Can you work these out from the model? Positions are in its coordinate system, mm. A direction names the side the tool comes from. Give positions to 0.01 mm unless a question says otherwise; leave off trailing zeros. Write each loop counter-clockwise with the first axis right and the second up, starting at its lowest first coordinate (ties: lowest second). Pieces come first, ordered by that corner, then holes.
1. Suppose I cut it at B-B (x = 0). Please give me the cut outline in (y, z), and give its area (3 significant figures).
2. On a 3-axis mill with a long thin cutter (end or side, diameter ignored), from which of +Z, -Z, +X, -X, +Y, -Y can I reach the whole of each face in a straight line? I mean faces 3 (the flat face through (38.6, 0.4, -19.9)), 4 (the cylindrical face through (-20.96, -16.56, -26.84)), 5 (the flat face through (-20.625, -2, -38)). Say none if no direction works.
3. If I drill on probe 1 along X at (y, z) = (-15, -34.1) (3 decimals); probe 2 along Y at (x, z) = (-16, -33); probe 3 along Y at (x, z) = (16, -27.5), over which ranges is the centre line in solid material (lowest first)?
4. Thinking about a two-plate mould opening in X: for faces 1 (the flat face through (32.35, 0.39, -13.32)), 2 (the cylindrical face through (32.097, 0.147, -14.115)), which applies, pulls with the +X half, pulls with the -X half, needs draft (parallel to the pull), parting line crosses it, or undercut?
5. Suppose I cut it at A-A (z = 0). Please give me the cut outline in (x, y), and give its area (3 significant figures).
6. Suppose I cut it at D-D (y = 8.5). Please give me the cut outline in (x, z) (1 decimal), and give its area (3 significant figures).
7. I'm going to push flat-ended pins straight in: pin 1 (7 mm diameter, centred on x = -16, y = -15, fed in from -Z); pin 2 (4 mm diameter, centred on x = 10.5, y = -6, fed in from +Z); pin 3 (10 mm diameter, centred on y = -12, z = 20.5, fed in from +X); pin 4 (13.5 mm diameter, centred on x = -16, y = -15, fed in from -Z). Where does each tip first touch, or does it pass through?
8. Suppose I cut it at C-C (x = 16). Please give me the cut outline in (y, z).
```python
from build123d import *

# Parameters (mm, degrees)
BOSS_EXTRUDE1_DEPTH                            = 27.5
CBORE_FOR_M3_SBHCS1_D                          = 3.4
CBORE_FOR_M3_SBHCS1_DEPTH                      = 20.0000108
CBORE_FOR_M3_SBHCS1_CBORE_D                    = 6.7
CBORE_FOR_M3_SBHCS1_CBORE_DEPTH                = 1.65
CBORE_FOR_M3_SBHCS1_TIP                        = 1.021463052
SKETCH4_W                                      = 41.25
SKETCH4_H                                      = 6.157842489
BOSS_EXTRUDE2_DEPTH                            = 4.5
CSK_FOR_M5_FLAT_HEAD_MACHINE_SCREW1_AT_2_COUNT = 2
CSK_FOR_M5_FLAT_HEAD_MACHINE_SCREW1_AT_2_PITCH = 32
CSK_FOR_M5_FLAT_HEAD_MACHINE_SCREW1_AT_3_COUNT = 2
CSK_FOR_M5_FLAT_HEAD_MACHINE_SCREW1_AT_3_PITCH = 43.863424399
CSK_FOR_M5_FLAT_HEAD_MACHINE_SCREW1_AT_4_COUNT = 2
CSK_FOR_M5_FLAT_HEAD_MACHINE_SCREW1_AT_4_PITCH = 30
CUT_EXTRUDE1_REACH                             = 81.852
CUT_EXTRUDE1_END_RADIUS                        = 30.1625
SKETCH13_R                                     = 5.2


with BuildPart() as part:
    # Sketch1 → Boss-Extrude1 (new, symmetric)
    with BuildSketch(Plane(origin=(0, 0, 0), x_dir=(1, 0, 0), z_dir=(0, 1, 0))):
        with BuildLine():
            Line((-25.625, 41.495342489), (-25.625, 21.324827813))
            ThreePointArc((-25.625, 21.324827813), (-5.163493362, -32.935197624), (30.921632796, 12.45959596))
            Line((30.921632796, 12.45959596), (39.848528412, 17.823415986))
            Line((39.848528412, 17.823415986), (37.273338038, 22.109252489))
            Line((37.273338038, 22.109252489), (28.701665031, 16.95887174))
            Line((28.701665031, 16.95887174), (28.843705147, 8.821398963))
            ThreePointArc((28.843705147, 8.821398963), (-27.915992451, -11.422511622), (26.75426667, 13.927872098))
            Line((26.75426667, 13.927872098), (26.647715613, 20.032178086))
            Line((26.647715613, 20.032178086), (35.371714531, 25.274085476))
            Line((35.371714531, 25.274085476), (32.281486081, 30.41708928))
            Line((32.281486081, 30.41708928), (23.557487163, 25.17518189))
            Line((23.557487163, 25.17518189), (20.982296789, 29.461018394))
            Line((20.982296789, 29.461018394), (29.706295707, 34.702925784))
            Line((29.706295707, 34.702925784), (25.625, 41.495342489))
            Line((25.625, 41.495342489), (20.625, 41.495342489))
            Line((20.625, 41.495342489), (20.625, 35.3375))
            Line((20.625, 35.3375), (-20.625, 35.3375))
            Line((-20.625, 35.3375), (-20.625, 41.495342489))
            Line((-20.625, 41.495342489), (-25.625, 41.495342489))
        make_face()
    extrude(amount=BOSS_EXTRUDE1_DEPTH, both=True)

    # CBORE for M3 SBHCS1
    with Locations(Plane(origin=(2.701817631, 0, 4.496579649), x_dir=(0.8571673007021098, 0, -0.5150380749100585), z_dir=(0.5150380749100585, 0, 0.8571673007021098))):
        with Locations((38.129386114, 20), (38.129386114, 0), (38.129386114, -20)):
            CounterBoreHole(CBORE_FOR_M3_SBHCS1_D / 2, CBORE_FOR_M3_SBHCS1_CBORE_D / 2, CBORE_FOR_M3_SBHCS1_CBORE_DEPTH, depth=CBORE_FOR_M3_SBHCS1_DEPTH)
            with Locations((0, 0, -(CBORE_FOR_M3_SBHCS1_DEPTH + CBORE_FOR_M3_SBHCS1_TIP / 2))):  # 118° drill point
                Cone(0, CBORE_FOR_M3_SBHCS1_D / 2, CBORE_FOR_M3_SBHCS1_TIP, mode=Mode.SUBTRACT)

    # Sketch4 → Boss-Extrude2 (add)
    with BuildSketch(Plane.XZ.offset(-27.5)):
        with Locations((0, -38.416421245)):
            Rectangle(SKETCH4_W, SKETCH4_H)
    extrude(amount=BOSS_EXTRUDE2_DEPTH)

    # Sketch12 → CSK for M5 Flat Head Machine Screw1 (revolve, cut)
    with BuildSketch(Plane(origin=(-16, 15, -30.1625), x_dir=(0, -1, 0), z_dir=(1, 0, 0))):
        Polygon((0, 0), (0, 11.332842489), (2.75, 11.332842489), (2.75, 2.45), (5.2, 0), align=None)
    csk_for_m5_flat_head_machine_screw1 = revolve(axis=Axis((-16, 15, -23.8125), (0, 0, -1)), mode=Mode.SUBTRACT)

    # CSK for M5 Flat Head Machine Screw1 at 2: CSK for M5 Flat Head Machine Screw1 ×2
    with Locations(*[(i * CSK_FOR_M5_FLAT_HEAD_MACHINE_SCREW1_AT_2_PITCH, 0, 0) for i in range(1, CSK_FOR_M5_FLAT_HEAD_MACHINE_SCREW1_AT_2_COUNT)]):
        add(csk_for_m5_flat_head_machine_screw1, mode=Mode.SUBTRACT)

    # CSK for M5 Flat Head Machine Screw1 at 3: CSK for M5 Flat Head Machine Screw1 ×2
    with Locations(*[Vector(0.7295372041400853, -0.6839411288813297, 0) * (i * CSK_FOR_M5_FLAT_HEAD_MACHINE_SCREW1_AT_3_PITCH) for i in range(1, CSK_FOR_M5_FLAT_HEAD_MACHINE_SCREW1_AT_3_COUNT)]):
        add(csk_for_m5_flat_head_machine_screw1, mode=Mode.SUBTRACT)

    # CSK for M5 Flat Head Machine Screw1 at 4: CSK for M5 Flat Head Machine Screw1 ×2
    with Locations(*[(0, -i * CSK_FOR_M5_FLAT_HEAD_MACHINE_SCREW1_AT_4_PITCH, 0) for i in range(1, CSK_FOR_M5_FLAT_HEAD_MACHINE_SCREW1_AT_4_COUNT)]):
        add(csk_for_m5_flat_head_machine_screw1, mode=Mode.SUBTRACT)

    # Cut-Extrude1: up to this cylinder (the profile starts outside it)
    cut_extrude1_end = Plane(origin=(0, 0, 0), z_dir=(0, -1, 0)) * Cylinder(CUT_EXTRUDE1_END_RADIUS, 255.029, mode=Mode.PRIVATE)
    # Sketch13 → Cut-Extrude1 (cut, up to the surface)
    with BuildSketch(Plane.XY.offset(-30.1625), mode=Mode.PRIVATE) as cut_extrude1_sk1:
        with Locations(Location((-16, -15, 0), (0, 0, 180))):
            Circle(SKETCH13_R)
    cut_extrude1_tool1 = extrude(cut_extrude1_sk1.sketch, amount=CUT_EXTRUDE1_REACH, mode=Mode.PRIVATE) - cut_extrude1_end
    add(cut_extrude1_tool1.solids().sort_by_distance((-16, -15, -30.1625))[0], mode=Mode.SUBTRACT)
    # Sketch13 → Cut-Extrude1 (cut, up to the surface)
    with BuildSketch(Plane.XY.offset(-30.1625), mode=Mode.PRIVATE) as cut_extrude1_sk2:
        with Locations(Location((16, -15, 0), (0, 0, 180))):
            Circle(SKETCH13_R)
    cut_extrude1_tool2 = extrude(cut_extrude1_sk2.sketch, amount=CUT_EXTRUDE1_REACH, mode=Mode.PRIVATE) - cut_extrude1_end
    add(cut_extrude1_tool2.solids().sort_by_distance((16, -15, -30.1625))[0], mode=Mode.SUBTRACT)
    # Sketch13 → Cut-Extrude1 (cut, up to the surface)
    with BuildSketch(Plane.XY.offset(-30.1625), mode=Mode.PRIVATE) as cut_extrude1_sk3:
        with Locations(Location((16, 15, 0), (0, 0, 180))):
            Circle(SKETCH13_R)
    cut_extrude1_tool3 = extrude(cut_extrude1_sk3.sketch, amount=CUT_EXTRUDE1_REACH, mode=Mode.PRIVATE) - cut_extrude1_end
    add(cut_extrude1_tool3.solids().sort_by_distance((16, 15, -30.1625))[0], mode=Mode.SUBTRACT)
    # Sketch13 → Cut-Extrude1 (cut, up to the surface)
    with BuildSketch(Plane.XY.offset(-30.1625), mode=Mode.PRIVATE) as cut_extrude1_sk4:
        with Locations(Location((-16, 15, 0), (0, 0, 180))):
            Circle(SKETCH13_R)
    cut_extrude1_tool4 = extrude(cut_extrude1_sk4.sketch, amount=CUT_EXTRUDE1_REACH, mode=Mode.PRIVATE) - cut_extrude1_end
    add(cut_extrude1_tool4.solids().sort_by_distance((-16, 15, -30.1625))[0], mode=Mode.SUBTRACT)


solid = part.part
```
Checks:
1. outline: (-27.5, -35.34) - (23, -35.34) - (23, -41.5) - (27.5, -41.5) - (27.5, -30.16) - (-27.5, -30.16) - close; (-27.5, 30.16) - (27.5, 30.16) - (27.5, 33.34) - (-27.5, 33.34) - close
1. area: 487 mm2
2. face 3: -Z, +X, +Y, -Y
2. face 4: none
2. face 5: -Z, -Y
3. probe 1: x = -25.625 to -18.75, -13.25 to 13.25, 18.75 to 28.703
3. probe 2: y = -27.5 to -17.75, -12.25 to 12.25, 17.75 to 27.5
3. probe 3: y = -27.5 to -20.2, -9.8 to 9.8, 20.2 to 27.5
4. face 1: pulls with the +X half
4. face 2: undercut
5. outline: (-33.34, -27.5) - (-30.16, -27.5) - (-30.16, 27.5) - (-33.34, 27.5) - close; (30.16, -27.5) - (33.34, -27.5) - (33.34, 27.5) - (30.16, 27.5) - close
5. area: 349 mm2
6. outline: (-25.6, -41.5) - (-20.6, -41.5) - (-20.6, -35.3) - (20.6, -35.3) - (20.6, -41.5) - (25.6, -41.5) - (29.7, -34.7) - (21, -29.5) - (23.6, -25.2) - (32.3, -30.4) - (35.4, -25.3) - (26.6, -20) - (26.8, -13.9) arc R30.2 cw (long way) to (28.8, -8.8) - (28.7, -17) - (37.3, -22.1) - (39.8, -17.8) - (30.9, -12.5) arc R33.3 ccw (long way) to (-25.6, -21.3) - close
6. area: 1,080 mm2
7. pin 1: stops at z = -35.34
7. pin 2: stops at z = 32.24
7. pin 3: stops at x = 29.52
7. pin 4: stops at z = -41.5
8. outline: (-27.5, -35.34) - (-17.75, -35.34) - (-17.75, -32.61) - (-20.2, -30.16) - (-20.2, -25.57) - (-27.5, -25.57) - close; (-27.5, 25.57) - (27.5, 25.57) - (27.5, 29.25) - (-27.5, 29.25) - close; (-12.25, -35.34) - (12.25, -35.34) - (12.25, -32.61) - (9.8, -30.16) - (9.8, -25.57) - (-9.8, -25.57) - (-9.8, -30.16) - (-12.25, -32.61) - close; (17.75, -35.34) - (23, -35.34) - (23, -41.5) - (27.5, -41.5) - (27.5, -25.57) - (20.2, -25.57) - (20.2, -30.16) - (17.75, -32.61) - close
